Build history of the part. All positions in model axes, mm. Give positions to 0.01 mm unless a question says otherwise; leave off trailing zeros. Loops run counter-clockwise (first coordinate to the right, second up) from the corner with the lowest first, then second, coordinate; pieces in that order, holes last. Notation, with made-up numbers: M 61.25,-23 L 94.25,-23 A28 ccw 94.25,-5 Z; hole C -1,71 d3. An arc over 180 degrees is marked long. Answer in a Markdown table with one row per item. Add a question column.
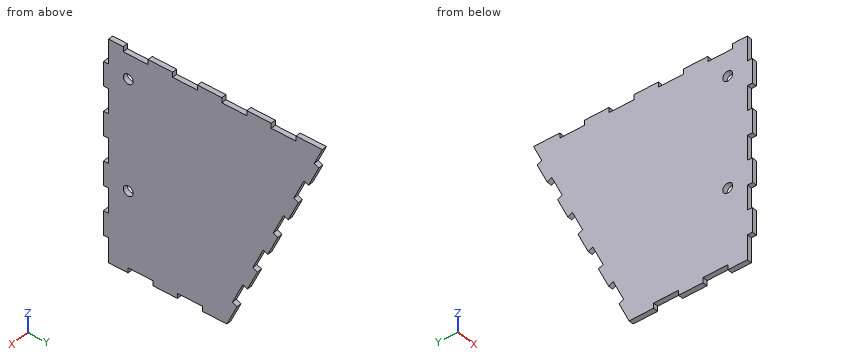
```python
from build123d import *

# Parameters (mm, degrees)
BOSS_EXTRUDE1_DEPTH = 4
SKETCH2_W           = 20.2
SKETCH2_H           = 4.1
CUT_EXTRUDE1_DEPTH  = 5
LPATTERN1_COUNT     = 6
LPATTERN1_PITCH     = 40
SKETCH3_W           = 4.1
SKETCH3_H           = 20.2
CUT_EXTRUDE2_DEPTH  = 4
LPATTERN2_COUNT     = 4
LPATTERN2_PITCH     = 40
SKETCH4_W           = 4.1
SKETCH4_H           = 20.2
CUT_EXTRUDE3_DEPTH  = 4
LPATTERN3_COUNT     = 2
LPATTERN3_PITCH     = 40
CUT_EXTRUDE4_DEPTH  = 4
LPATTERN4_COUNT     = 6
LPATTERN4_PITCH     = 40
SKETCH6_R           = 4
CUT_EXTRUDE5_DEPTH  = 5


with BuildPart() as part:
    # Sketch1 → Boss-Extrude1 (new body)
    with BuildSketch(Plane(origin=(0, 0, 0), x_dir=(0, 0, -1), z_dir=(1, 0, 0))):
        Polygon((-60.155879739, 92), (119.844120261, 10), (119.844120261, -90), (-60.155879739, -90), align=None)
    extrude(amount=BOSS_EXTRUDE1_DEPTH)

    # Sketch2 → Cut-Extrude1 (cut, through all)
    with BuildSketch(Plane(origin=(4, 0, 0), x_dir=(0, 0, -1), z_dir=(1, 0, 0))):
        with Locations((-50.155879739, -87.95)):
            Rectangle(SKETCH2_W, SKETCH2_H)
    cut_extrude1 = extrude(amount=-CUT_EXTRUDE1_DEPTH, mode=Mode.SUBTRACT)

    # LPattern1: Cut-Extrude1 ×6
    with Locations(*[(0, 0, -i * LPATTERN1_PITCH) for i in range(1, LPATTERN1_COUNT)]):
        add(cut_extrude1, mode=Mode.SUBTRACT)

    # Sketch3 → Cut-Extrude2 (cut)
    with BuildSketch(Plane(origin=(4, 0, 0), x_dir=(0, 0, -1), z_dir=(1, 0, 0))):
        with Locations((-58.105879739, -63.9)):
            Rectangle(SKETCH3_W, SKETCH3_H)
    cut_extrude2 = extrude(amount=-CUT_EXTRUDE2_DEPTH, mode=Mode.SUBTRACT)

    # LPattern2: Cut-Extrude2 ×4
    with Locations(*[(0, i * LPATTERN2_PITCH, 0) for i in range(1, LPATTERN2_COUNT)]):
        add(cut_extrude2, mode=Mode.SUBTRACT)

    # Sketch4 → Cut-Extrude3 (cut)
    with BuildSketch(Plane(origin=(4, 0, 0), x_dir=(0, 0, -1), z_dir=(1, 0, 0))):
        with Locations((117.794120261, -60)):
            Rectangle(SKETCH4_W, SKETCH4_H)
    cut_extrude3 = extrude(amount=-CUT_EXTRUDE3_DEPTH, mode=Mode.SUBTRACT)

    # LPattern3: Cut-Extrude3 ×2
    with Locations(*[(0, i * LPATTERN3_PITCH, 0) for i in range(1, LPATTERN3_COUNT)]):
        add(cut_extrude3, mode=Mode.SUBTRACT)

    # Sketch5 → Cut-Extrude4 (cut)
    with BuildSketch(Plane(origin=(4, 0, 0), x_dir=(0, 0, -1), z_dir=(1, 0, 0))):
        Polygon((101.734724645, 18.249835781), (83.352323065, 26.624040945), (81.652608155, 22.892959436), (100.035009735, 14.518754272), align=None)
    cut_extrude4 = extrude(amount=-CUT_EXTRUDE4_DEPTH, mode=Mode.SUBTRACT)

    # LPattern4: Cut-Extrude4 ×6
    with Locations(*[Vector(0, 0.414564612, 0.91001988) * (i * LPATTERN4_PITCH) for i in range(1, LPATTERN4_COUNT)]):
        add(cut_extrude4, mode=Mode.SUBTRACT)

    # Sketch6 → Cut-Extrude5 (cut, through all)
    with BuildSketch(Plane(origin=(4, 0, 0), x_dir=(0, 0, -1), z_dir=(1, 0, 0))):
        with Locations((-36.055879739, -70)):
            Circle(SKETCH6_R)
        with Locations((53.944120261, -70)):
            Circle(SKETCH6_R)
    extrude(amount=-CUT_EXTRUDE5_DEPTH, mode=Mode.SUBTRACT)


solid = part.part
```
(1) Slice it at C-C, the plane y = -63.5. Give the cut face in (x, z).
(2) Wall check: line 1 (Z direction, x = 1.55, y = 70.5); line 2 (Z direction, x = 0.8, y = -33); line 3 (Z direction, x = 1.5, y = -69). Give the ranges that are in metal, low to high.
(3) Slice it at B-B, the plane x = 2.35. State how many separate pieces and enclosed holes the cut face has, then the cut area to 3 significant figures.
(4) Pin check, flat tips, straight feed: pin 1 (2 mm diameter, centred on x = 1.5, z = -118.5, fed in from +Y); pin 2 (2 mm diameter, centred on x = 2.5, y = -87.5, fed in from -Z); pin 3 (1.2 mm diameter, centred on x = 2, z = 59, fed in from +Y). Stop position of each tip, or through.
(5) Slice it at D-D, the plane z = -6.5. Give the cut face in (x, y), then the cut area to 3 significant figures.
(6) Slice it at A-A, the plane z = -54. Give the cut face in (x, y).
Solution:
| question | item | result |
|---|---|---|
| 1 | outline | M 0,-115.74 L 4,-115.74 L 4,56.06 L 0,56.06 Z |
| 2 | line 1 | 22.85 to 60.16 |
| 2 | line 2 | -119.84 to 56.06 |
| 2 | line 3 | -115.74 to -57.82, -50.07 to 32.18, 39.93 to 56.06 |
| 3 | separate pieces | 1 |
| 3 | enclosed holes | 2 |
| 3 | area | 24,000 mm^2 |
| 4 | pin 1 | y = 11.07 |
| 4 | pin 2 | z = -99.74 |
| 4 | pin 3 | y = 87.24 |
| 5 | outline | M 0,-90 L 4,-90 L 4,61.63 L 0,61.63 Z |
| 5 | area | 607 mm^2 |
| 6 | outline | M 0,-90 L 4,-90 L 4,-74 L 0,-74 Z; M 0,-66 L 4,-66 L 4,35.49 L 0,35.49 Z |
